Input: dimensioned drawing with shaded views. Units: mm. Origin: part minimum x, y, z. Give positions to 0.01 mm unless a question says otherwise; leave off trailing zeros. Order: outer loops, then holes, each group sorted by start corner. A loop starts at its lowest first (then second) coordinate and runs counter-clockwise, first axis right, second up.
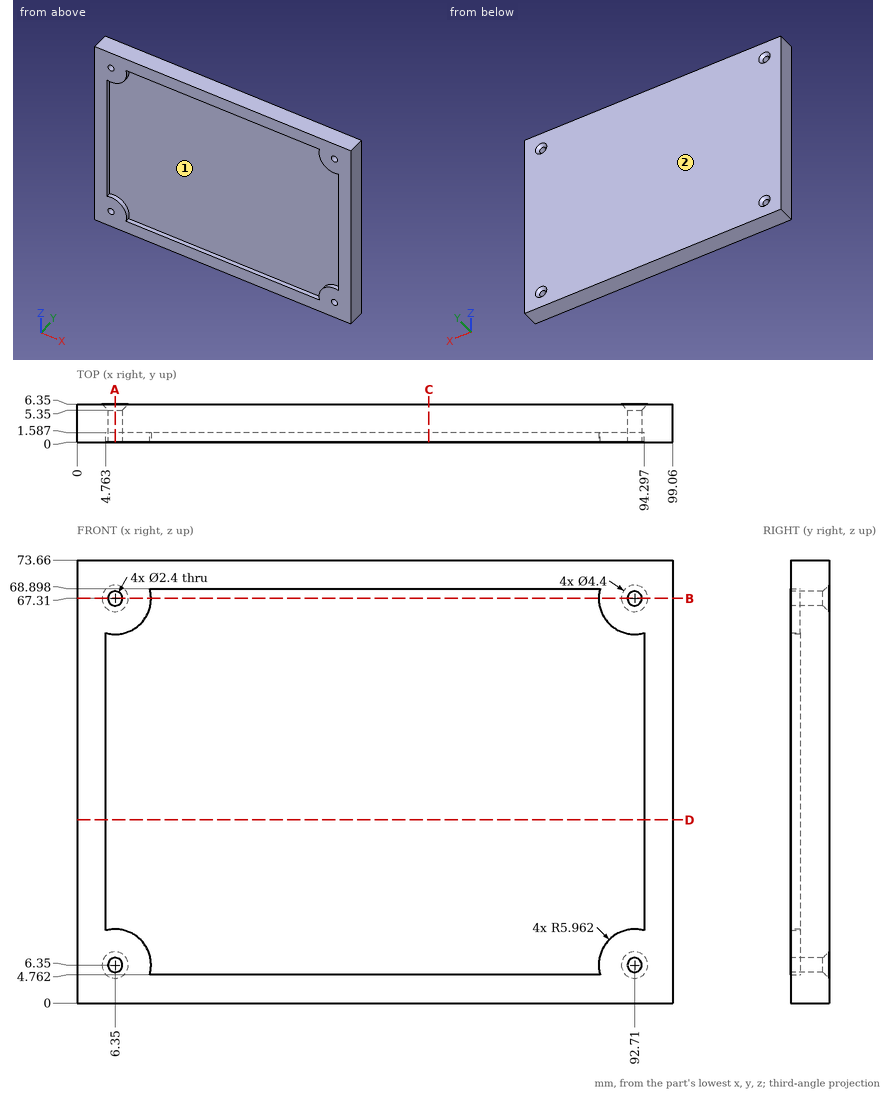
1) Cut plane A-A (x = 6.35). Return the cut outline in (y, z).
2) Cut plane D-D (z = 30.5). Return the cut outline in (x, y), then the cut area to 3 significant figures.
3) Cut plane B-B (z = 67.31). Return the cut outline in (x, y).
4) Cut plane C-C (x = 58.5). Return the cut outline in (y, z), then the cut area to 3 significant figures.
5) First-contact query: P1, Ø2, axis at x = 6.35, z = 6.35, coming from the -Y side; P2, Ø10, axis at x = 38.5, z = 32, coming from the -Y side; P3, Ø4, axis at x = 92.71, z = 6.35, coming from the +Y side. Flat tips, straight axial feed; report the tip coordinate or a pass-through.
6) Pull-direction query (Z, two-part tool) for the marked faces 1 and 2; classes: pulls with the +Z half, pulls with the -Z half, needs draft (parallel to the pull), parting line crosses it, or undercut.
7) Line query: probe 1 along X at (y, z) = (2.85, 6.35); probe 2 along X at (y, z) = (1.25, 6.35); probe 3 along Z at (x, y) = (92.71, 4). Output: solid intervals per line, ascending.
Geometry says:
1. outline: (0, 0) - (6.35, 0) - (6.35, 4.15) - (5.35, 5.15) - (0, 5.15) - close; (0, 7.55) - (5.35, 7.55) - (6.35, 8.55) - (6.35, 65.11) - (5.35, 66.11) - (0, 66.11) - (0, 61.35) - (1.59, 61.35) - (1.59, 12.31) - (0, 12.31) - close; (0, 68.51) - (5.35, 68.51) - (6.35, 69.51) - (6.35, 73.66) - (0, 73.66) - close
2. outline: (0, 0) - (4.76, 0) - (4.76, 1.59) - (94.3, 1.59) - (94.3, 0) - (99.06, 0) - (99.06, 6.35) - (0, 6.35) - close
2. area: 487 mm2
3. outline: (0, 0) - (5.15, 0) - (5.15, 5.35) - (4.15, 6.35) - (0, 6.35) - close; (7.55, 0) - (12.31, 0) - (12.31, 1.59) - (86.75, 1.59) - (86.75, 0) - (91.51, 0) - (91.51, 5.35) - (90.51, 6.35) - (8.55, 6.35) - (7.55, 5.35) - close; (93.91, 0) - (99.06, 0) - (99.06, 6.35) - (94.91, 6.35) - (93.91, 5.35) - close
4. outline: (0, 0) - (6.35, 0) - (6.35, 73.66) - (0, 73.66) - (0, 68.9) - (1.59, 68.9) - (1.59, 4.76) - (0, 4.76) - close
4. area: 366 mm2
5. P1: passes through
5. P2: stops at y = 1.59
5. P3: stops at y = 6.15
6. face 1: undercut
6. face 2: needs draft
7. probe 1: x = 0 to 5.15, 7.55 to 91.51, 93.91 to 99.06
7. probe 2: x = 0 to 5.15, 7.55 to 12.31, 86.75 to 91.51, 93.91 to 99.06
7. probe 3: z = 0 to 5.15, 7.55 to 66.11, 68.51 to 73.66
